Check sheet for the modelled part. Datum: model origin and axes. Units: mm. A direction names the side the tool comes from. Give positions to 0.01 mm unless a question says otherwise; leave off trailing zeros. Write each loop counter-clockwise with the first axis right and the second up, starting at its lowest first coordinate (ties: lowest second). Pieces come first, ordered by that corner, then holes. Notation, with made-up numbers: M 4.5,76 L 41.5,76 A28 ccw 41.5,102 Z; hole C -36.75,89.25 d8. An arc over 180 degrees is marked long. Write item = value, one per line. Start each with the question number.
1) Cross-section at B-B, the plane x = -23.5. Record the cut outline in (y, z), plus the area to 3 significant figures.
2) Access from +Z, -Z, +X, -X, +Y, -Y to the whole of each face (thin tool, end or side, straight path). Record for faces 1 (the flat face through (-29.7, 81.6, 3.1)), 2 (the flat face through (5, 95, 6.35)), 3 (the flat face through (0, 165, 3)).
3) Cross-section at D-D, the plane y = 183.5. Record the cut outline in (x, z), plus the area to 3 significant figures.
4) Go/stop test with flat-tipped pins: pin 1 (3 mm diameter, centred on x = -2.5, y = 73, fed in from +Z); pin 2 (1.9 mm diameter, centred on y = 126.5, z = 3, fed in from +X). Record where each tip stops, or that it passes through.
5) Mould release check, pull along Y, two halves, no side actions. Record for faces 4 (the cylindrical face through (9.68, 194.205, 3.219)), 5 (the flat face through (63.46, 90.63, 3.13)), 6 (the flat face through (-57.576, 158.19, 3.131)): released by +Y, released by -Y, zero draft, split by the parting line, or undercut.
6) Scan lines: line 1 along Y through (x, z) = (10.16, 3.5); line 2 along X through (y, z) = (69, 5.5); line 3 along X through (y, z) = (49, 4.5). Record each from-to range of solid material in increasing order. Write a range as [from, to].
7) Cross-section at A-A, the plane y = 0. Record the cut outline in (x, z) (3 decimals), plus the area to 3 significant figures.
8) Cross-section at C-C, the plane z = 1.25. Give the number of separate pieces and of enclosed holes in the cut face, plus the area to 3 significant figures.
```python
from build123d import *

# Parameters (mm, degrees)
SKETCH1_R          = 3.175
BASE_EXTRUDE_DEPTH = 6.35
FILLET1_R          = 10
FILLET2_R          = 2.54
SKETCH2_R          = 2.54
MOUNT_HOLES_DEPTH  = 233.825979653
FILLET3_R          = 25.24


with BuildPart() as part:
    # Sketch1 → Base Extrude (new body)
    with BuildSketch(Plane.XY):
        with BuildLine():
            Line((-75.671499827, 189.250953956), (-10.702976856, 8.978150501))
            ThreePointArc((-10.702976856, 8.978150501), (1.824481313, -13.850349019), (8.012862816, 11.443554059))
            Line((8.012862816, 11.443554059), (116.905655655, 166.9585791))
            ThreePointArc((116.905655655, 166.9585791), (61.289492424, 194.385435611), (0, 203.818790741))
            Line((0, 203.818790741), (0, 136.3309927))
            ThreePointArc((0, 136.3309927), (-19.864532894, 112.657364258), (-46.627945663, 128.109227825))
            Line((-46.627945663, 128.109227825), (-69.710132022, 191.527013637))
            ThreePointArc((-69.710132022, 191.527013637), (-72.699723739, 190.4123148), (-75.671499827, 189.250953956))
        make_face()
        Circle(SKETCH1_R, mode=Mode.SUBTRACT)
        with BuildLine():
            Line((26.680843247, 49.175080254), (108.003253412, 165.315518235))
            ThreePointArc((108.003253412, 165.315518235), (59.380010597, 188.329332974), (6.35, 197.366665921))
            Line((6.35, 197.366665921), (6.35, 55.585370506))
            ThreePointArc((6.35, 55.585370506), (14.165311985, 44.926629865), (26.680843247, 49.175080254))
        make_face(mode=Mode.SUBTRACT)
        with BuildLine():
            Line((0, 55.102439922), (0, 117.740251175))
            ThreePointArc((0, 117.740251175), (-18.761866966, 106.403835026), (-40.269537582, 110.639645198))
            Line((-40.269537582, 110.639645198), (-18.8461444, 51.779356182))
            ThreePointArc((-18.8461444, 51.779356182), (-8.02887303, 45.534001644), (0, 55.102439922))
        make_face(mode=Mode.SUBTRACT)
    extrude(amount=BASE_EXTRUDE_DEPTH)

    # Fillet1
    fillet1_edges = [part.edges().sort_by_distance(p)[0] for p in [
        (0, 203.818790741, 3.175),
        (116.905655655, 166.9585791, 3.175),
        (108.003253412, 165.315518235, 3.175),
        (6.35, 197.366665921, 3.175),
    ]]
    fillet(fillet1_edges, radius=FILLET1_R)

    # Fillet2
    fillet2_edges = [part.edges().sort_by_distance(p)[0] for p in [
        (-75.671499827, 189.250953956, 3.175),
        (-69.710132022, 191.527013637, 3.175),
    ]]
    fillet(fillet2_edges, radius=FILLET2_R)

    # Sketch2 → Mount Holes (cut, through all)
    with BuildSketch(Plane.XY.offset(6.35)):
        with Locations((0, 10.16)):
            Circle(SKETCH2_R)
        with Locations((10.16, 0)):
            Circle(SKETCH2_R)
        with Locations((0, -10.16)):
            Circle(SKETCH2_R)
        with Locations((-10.16, 0)):
            Circle(SKETCH2_R)
    extrude(amount=-MOUNT_HOLES_DEPTH, mode=Mode.SUBTRACT)

    # Fillet3
    fillet3_edges = [part.edges().sort_by_distance(p)[0] for p in [
        (8.012862816, 11.443554059, 3.175),
        (-10.702976856, 8.978150501, 3.175),
    ]]
    fillet(fillet3_edges, radius=FILLET3_R)


solid = part.part
```
Reply:
q1.outline = M 44.49,0 L 64.57,0 L 64.57,6.35 L 44.49,6.35 Z; M 105.95,0 L 112.3,0 L 112.3,6.35 L 105.95,6.35 Z
q1.area = 168 mm2
q2.face_1 = +Z, -Z
q2.face_2 = +Z, +X, -X, +Y, -Y
q2.face_3 = +Z, -Z, +Y
q3.outline = M -73.6,0 L -66.79,0 L -66.79,6.35 L -73.6,6.35 Z; M 0,0 L 6.35,0 L 6.35,6.35 L 0,6.35 Z; M 72.95,0 L 88.71,0 L 88.71,6.35 L 72.95,6.35 Z
q3.area = 184 mm2
q4.pin_1 = through
q4.pin_2 = 89.24
q5.face_4 = undercut
q5.face_5 = released by -Y
q5.face_6 = released by +Y
q6.line_1 = [-9.59, -2.54], [2.54, 47.18], [194.61, 203.56]
q6.line_2 = [-32.33, -25.11], [0, 6.35], [40.56, 48.31]
q6.line_3 = [-25.13, -17.28], [-2.16, 8.5], [26.56, 34.31]
q7.outline = M -13.97,0 L -12.7,0 L -12.7,6.35 L -13.97,6.35 Z; M -7.62,0 L -3.175,0 L -3.175,6.35 L -7.62,6.35 Z; M 3.175,0 L 7.62,0 L 7.62,6.35 L 3.175,6.35 Z; M 12.7,0 L 13.97,0 L 13.97,6.35 L 12.7,6.35 Z
q7.area = 72.6 mm2
q8.separate_pieces = 1
q8.enclosed_holes = 7
q8.area = 5,840 mm2
